Part model, mm, in its own coordinate system. Round coordinates to 2 decimals unless told otherwise and drop trailing zeros. Write each loop counter-clockwise with the first axis right and the second up, starting at its lowest first coordinate (ties: lowest second). Pieces come first, ordered by that corner, then holes. Notation, with made-up numbers: M -9.75,38 L 15.25,38 A5 cw 15.25,45 Z; hole C -22.75,82 d11. An arc over 180 degrees is marked long. Answer as a JSON object with one key per item and string values. Group by question number.
1. Band-saw the part on B-B, the plane y = 13. Write the cut outline in (x, z), plus the area to 3 significant figures.
2. Band-saw the part on C-C, the plane x = -5. Write the cut outline in (y, z).
3. Band-saw the part on A-A, the plane z = 3.4. Write the cut outline in (x, y), plus the area to 3 significant figures.
4. Drill centre lines: line 1 (Y direction, x = -4, z = 1.75); line 2 (X direction, y = 20, z = 0.65); line 3 (Z direction, x = 23, y = 15). Where is each one in solid material? Low to high. Write a range as from..to.
5. Drop flat-ended pins along their axis: pin 1 (1.7 mm diameter, centred on y = 25, z = 3.5, fed in from -X); pin 2 (3 mm diameter, centred on x = -9, y = 22, fed in from -Z); pin 3 (1.1 mm diameter, centred on x = 26.5, z = 3.5, fed in from -Y); pin 4 (1 mm diameter, centred on x = -11.5, z = 3, fed in from -Y). Give the stop position or say it passes through.
6. Band-saw the part on D-D, the plane x = 16.5. Write the cut outline in (y, z), plus the area to 3 significant figures.
from build123d import *

# Parameters (mm, degrees)
F1_DEPTH = 4.318
F0_W     = 60.96
F0_H     = 71.12
F0_W_2   = 54.61
F0_H_2   = 12.065
F0_W_3   = 3.81
F0_H_3   = 3.81
F2_DEPTH = 2.159
F3_R     = 5.08


with BuildPart() as f1:
    # F0 (on Top) → F1 (new body)
    with BuildSketch(Plane.XY):
        Polygon((-10.2077507393, 20.6597218627), (-20.3677507393, 30.8197218627), (-20.3677507393, 20.6597218627), align=None)
        Polygon((-10.2077507393, 20.6597218627), (-20.3677507393, 20.6597218627), (-20.3677507393, 10.4997218627), align=None)
        Polygon((-10.2077507393, 10.4997218627), (-10.2077507393, 20.6597218627), (-20.3677507393, 10.4997218627), align=None)
        Polygon((-10.2077507393, 10.4997218627), (-20.3677507393, 10.4997218627), (-10.2077507393, 0.3397218627), align=None)
        Polygon((-0.0477507393, 10.4997218627), (-10.2077507393, 10.4997218627), (-10.2077507393, 0.3397218627), (10.1122492607, 0.3397218627), align=None)
    extrude(amount=F1_DEPTH)



with BuildPart() as f1b:
    # F0 (on Top) → F1, piece 2 (new body)
    with BuildSketch(Plane.XY):
        Polygon((-0.0477507393, 30.8197218627), (-10.2077507393, 30.8197218627), (-0.0477507393, 20.6597218627), align=None)
        Polygon((10.1122492607, 20.6597218627), (-0.0477507393, 30.8197218627), (-0.0477507393, 20.6597218627), (3.7622492607, 20.6597218627), (6.3022492607, 20.6597218627), align=None)
        Polygon((10.1122492607, 30.8197218627), (-0.0477507393, 30.8197218627), (10.1122492607, 20.6597218627), align=None)
        Polygon((20.2722492607, 20.6597218627), (10.1122492607, 30.8197218627), (10.1122492607, 20.6597218627), align=None)
        Polygon((20.2722492607, 20.6597218627), (10.1122492607, 20.6597218627), (10.1122492607, 16.8497218627), (10.1122492607, 14.3097218627), (10.1122492607, 10.4997218627), (20.2722492607, 0.3397218627), (30.4322492607, 0.3397218627), (20.2722492607, 10.4997218627), align=None)
    extrude(amount=F1_DEPTH)


with BuildPart() as f1_1:
    add(f1.part)

    add(f1b.part)  # F2 merges F1b
    # F0 (on Top) → F2 (join)
    with BuildSketch(Plane.XY):
        with Locations((5.0322492607, 15.5797218627)):
            Rectangle(F0_W, F0_H)
        Polygon((-20.3677507393, 20.6597218627), (-20.3677507393, 30.8197218627), (-10.2077507393, 20.6597218627), (-10.2077507393, 10.4997218627), (-0.0477507393, 10.4997218627), (10.1122492607, 0.3397218627), (-10.2077507393, 0.3397218627), (-20.3677507393, 10.4997218627), align=None, mode=Mode.SUBTRACT)
        with Locations((5.0322492607, -10.7727781373)):
            Rectangle(F0_W_2, F0_H_2, mode=Mode.SUBTRACT)
        with Locations((5.0322492607, 41.9322218627)):
            Rectangle(F0_W_2, F0_H_2, mode=Mode.SUBTRACT)
        Polygon((-0.0477507393, 20.6597218627), (-10.2077507393, 30.8197218627), (-0.0477507393, 30.8197218627), (10.1122492607, 30.8197218627), (20.2722492607, 20.6597218627), (20.2722492607, 10.4997218627), (30.4322492607, 0.3397218627), (20.2722492607, 0.3397218627), (10.1122492607, 10.4997218627), (10.1122492607, 14.3097218627), (6.3022492607, 14.3097218627), (6.3022492607, 10.4997218627), (3.7622492607, 10.4997218627), (3.7622492607, 14.3097218627), (-0.0477507393, 14.3097218627), (-0.0477507393, 16.8497218627), (3.7622492607, 16.8497218627), (3.7622492607, 20.6597218627), align=None, mode=Mode.SUBTRACT)
        with Locations((8.2072492607, 18.7547218627)):
            Rectangle(F0_W_3, F0_H_3)
    extrude(amount=F2_DEPTH)

    # F3
    f3_edges = [f1_1.edges().sort_by_distance(p)[0] for p in [
        (-25.447751, -19.980278, 1.0795),
        (35.512249, -19.980278, 1.0795),
        (35.512249, 51.139722, 1.0795),
        (-25.447751, 51.139722, 1.0795),
        (-22.272751, -16.805278, 1.0795),
        (-22.272751, -4.740278, 1.0795),
        (-22.272751, 47.964722, 1.0795),
        (-22.272751, 35.899722, 1.0795),
        (32.337249, -16.805278, 1.0795),
        (32.337249, 35.899722, 1.0795),
        (32.337249, 47.964722, 1.0795),
        (32.337249, -4.740278, 1.0795),
    ]]
    fillet(f3_edges, radius=F3_R)


solid = f1_1.part
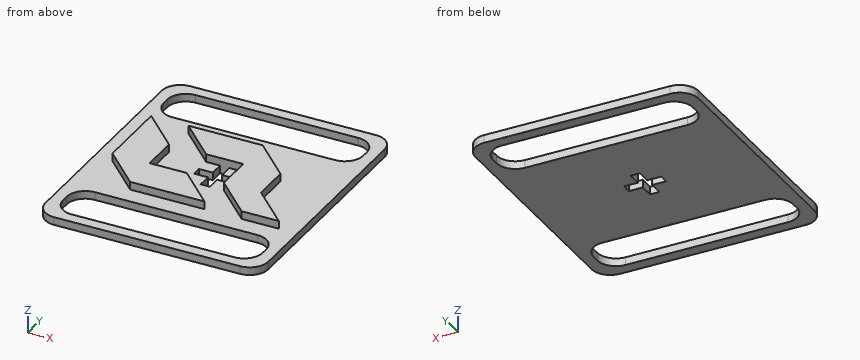
Worked answers:
{
 "1": {"outline": "M -25.45,0 L 3.76,0 L 3.76,2.16 L -10.21,2.16 L -10.21,4.32 L -20.37,4.32 L -20.37,2.16 L -25.45,2.16 Z; M 6.3,0 L 35.51,0 L 35.51,2.16 L 20.27,2.16 L 20.27,4.32 L 10.11,4.32 L 10.11,2.16 L 6.3,2.16 Z", "area": "170 mm^2"},
 "2": {"outline": "M -19.98,0 L -16.81,0 L -16.81,2.16 L -19.98,2.16 Z; M -4.74,0 L 35.9,0 L 35.9,2.16 L 30.82,2.16 L 30.82,4.32 L 25.61,4.32 L 25.61,2.16 L 10.5,2.16 L 10.5,4.32 L 0.34,4.32 L 0.34,2.16 L -4.74,2.16 Z; M 47.96,0 L 51.14,0 L 51.14,2.16 L 47.96,2.16 Z"},
 "3": {"outline": "M -20.37,10.5 L -10.21,0.34 L 10.11,0.34 L -0.05,10.5 L -10.21,10.5 L -10.21,20.66 L -20.37,30.82 Z; M -10.21,30.82 L -0.05,20.66 L 10.11,20.66 L 10.11,10.5 L 20.27,0.34 L 30.43,0.34 L 20.27,10.5 L 20.27,20.66 L 10.11,30.82 Z", "area": "774 mm^2"},
 "4": {"line 1": "y = -19.98..-16.81, -4.74..35.9, 47.96..51.14", "line 2": "x = -25.45..3.76, 6.3..35.51", "line 3": "z = 0..2.16"},
 "5": {"pin 1": "stops at x = -20.37", "pin 2": "stops at z = 0", "pin 3": "stops at y = 0.34", "pin 4": "stops at y = 1.13"},
 "6": {"outline": "M -19.98,0 L -16.81,0 L -16.81,2.16 L -19.98,2.16 Z; M -4.74,0 L 35.9,0 L 35.9,2.16 L 24.43,2.16 L 24.43,4.32 L 4.11,4.32 L 4.11,2.16 L -4.74,2.16 Z; M 47.96,0 L 51.14,0 L 51.14,2.16 L 47.96,2.16 Z", "area": "145 mm^2"}
}
